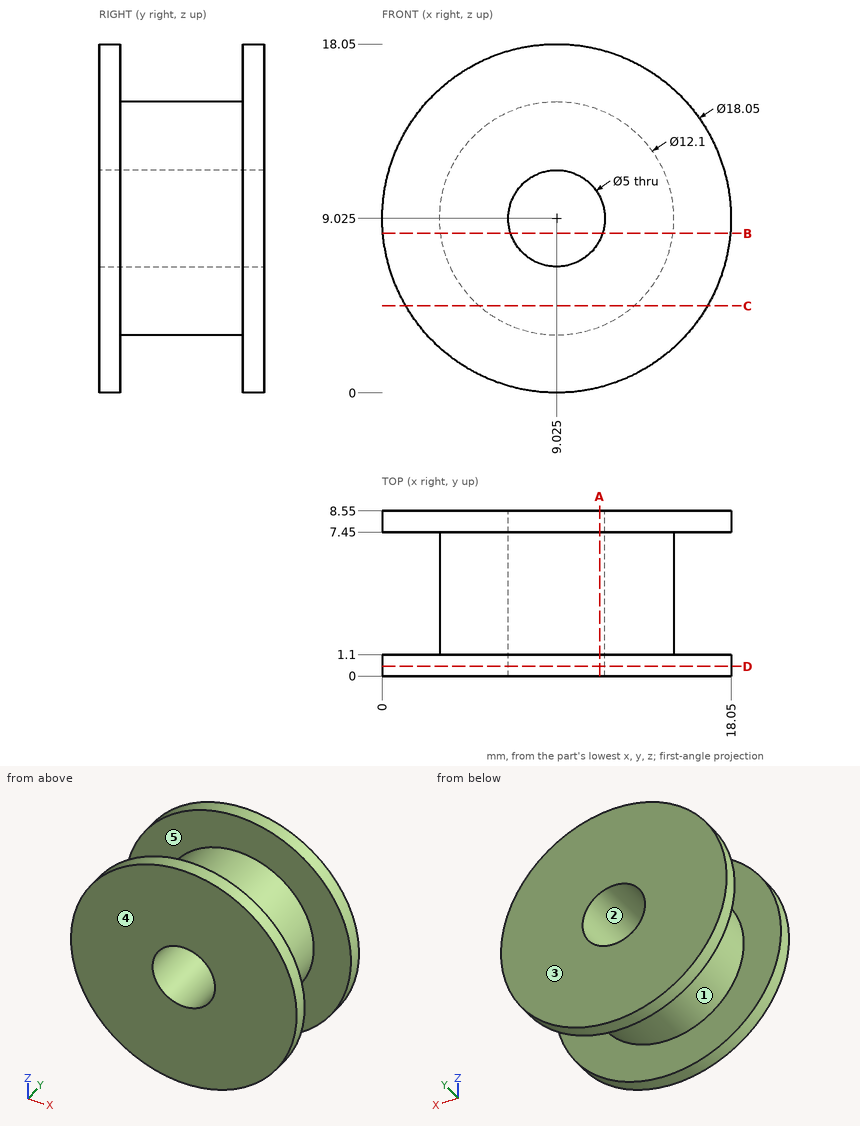
Source: three-view drawing plus pictorial views. Frame: mm from the lowest corner of the part. A direction names the side the tool comes from. Give positions to 0.01 mm unless a question says otherwise; leave off trailing zeros. Order: outer loops, then holes, each group sorted by start corner. A loop starts at its lowest first (then second) coordinate and runs counter-clockwise, first axis right, second up. Notation, with made-up numbers: (-17, 12.25) - (36, 12.25) arc R27 cw to (36, 35.25) - close; hole circle Ø6 at (6.5, -33). An arc over 180 degrees is marked (long way). Put each result on its own line as item: value.
Item 1: Ray query, L1, parallel to Y at x = 15.75, z = 12; L2, parallel to X at y = 2, z = 7.75; L3, parallel to X at y = 6, z = 10.5. Return the intervals inside material, ascending. Write a range as from..to.
Found:
L1: y = 0..1.1, 7.45..8.55
L2: x = 3.11..6.87, 11.18..14.94
L3: x = 3.16..7.01, 11.04..14.89
Item 2: Access query for the marked faces 1 and 2. Directions: +Z, -Z, +X, -X, +Y, -Y. A direction counts if a zero-diameter tool reaches every point of the face in a straight line with its end or side. Return the directions, or none.
Found:
face 1: none
face 2: +Y, -Y
Item 3: Section query C-C, the plane z = 4.5. Return loops of the section in (x, y).
Found:
outline: (1.22, 0) - (16.83, 0) - (16.83, 1.1) - (13.04, 1.1) - (13.04, 7.45) - (16.83, 7.45) - (16.83, 8.55) - (1.22, 8.55) - (1.22, 7.45) - (5.01, 7.45) - (5.01, 1.1) - (1.22, 1.1) - close
Item 4: Contact query for flat-ended pins moving along their axis: pin 1 (5 mm diameter, centred on x = 13, y = 2, fed in from +Z); pin 2 (1 mm diameter, centred on y = 5, z = 3, fed in from +X); pin 3 (1.5 mm diameter, centred on y = 1.5, z = 8, fed in from -X). Output: stop coordinate, or through.
Found:
pin 1: stops at z = 17.9
pin 2: stops at x = 11.49
pin 3: stops at x = 0.01
Item 5: Section query D-D, the plane y = 0.5. Return loops of the section in (x, z) (3 decimals), then the cut area to 3 significant figures.
Found:
outline: circle Ø18.05 at (9.025, 9.025); hole circle Ø5 at (9.025, 9.025)
area: 236 mm^2
Item 6: Draft query along Y for the marked faces 3, 4 and 5. Return one class per face: +Y half, -Y half, draft (parallel to the pull), parting line (faces both ways), or undercut.
Found:
face 3: +Y half
face 4: -Y half
face 5: undercut
Item 7: Section query A-A, the plane x = 11.25. Return loops of the section in (y, z), then the cut area to 3 significant figures.
Found:
outline: (0, 0.28) - (1.1, 0.28) - (1.1, 3.4) - (7.45, 3.4) - (7.45, 0.28) - (8.55, 0.28) - (8.55, 7.89) - (0, 7.89) - close; (0, 10.16) - (8.55, 10.16) - (8.55, 17.77) - (7.45, 17.77) - (7.45, 14.65) - (1.1, 14.65) - (1.1, 17.77) - (0, 17.77) - close
area: 90.4 mm^2
Item 8: Section query B-B, the plane z = 8.25. Return loops of the section in (x, y).
Found:
outline: (0.03, 0) - (6.65, 0) - (6.65, 8.55) - (0.03, 8.55) - (0.03, 7.45) - (3.02, 7.45) - (3.02, 1.1) - (0.03, 1.1) - close; (11.4, 0) - (18.02, 0) - (18.02, 1.1) - (15.03, 1.1) - (15.03, 7.45) - (18.02, 7.45) - (18.02, 8.55) - (11.4, 8.55) - close
